```python
from build123d import *

# Parameters (mm, degrees)
SKETCH_1_R      = 2
SKETCH_1_R_2    = 5.02
SKETCH_1_R_3    = 2.05
SKETCH_1_W      = 8.2
SKETCH_1_H      = 2.2
EXTRUDE_1_DEPTH = 2
FILLET_1_R      = 1


with BuildPart() as part:
    # 草图1 → 凸台-拉伸1 (new body)
    with BuildSketch(Plane.XY):
        with BuildLine():
            Line((-38.25, 66.25), (-38.25, 62.25))
            Line((-38.25, 62.25), (-40.15, 62.25))
            Line((-40.15, 62.25), (-40.15, 59.05))
            Line((-40.15, 59.05), (-38.25, 59.05))
            Line((-38.25, 59.05), (-38.25, 55.85))
            Line((-38.25, 55.85), (-34.15, 55.85))
            Line((-34.15, 55.85), (-34.15, 59.05))
            Line((-34.15, 59.05), (-32.25, 59.05))
            Line((-32.25, 59.05), (-32.25, 62.25))
            Line((-32.25, 62.25), (-34.15, 62.25))
            Line((-34.15, 62.25), (-34.15, 66.25))
            Line((-34.15, 66.25), (-25.2, 66.25))
            Line((-25.2, 66.25), (-25.2, 70.25))
            Line((-25.2, 70.25), (-17.2, 70.25))
            Line((-17.2, 70.25), (-17.2, 66.25))
            Line((-17.2, 66.25), (-8.25, 66.25))
            Line((-8.25, 66.25), (-8.25, 62.25))
            Line((-8.25, 62.25), (-10.15, 62.25))
            Line((-10.15, 62.25), (-10.15, 59.05))
            Line((-10.15, 59.05), (-8.25, 59.05))
            Line((-8.25, 59.05), (-8.25, 55.85))
            Line((-8.25, 55.85), (-4.15, 55.85))
            Line((-4.15, 55.85), (-4.15, 59.05))
            Line((-4.15, 59.05), (-2.25, 59.05))
            Line((-2.25, 59.05), (-2.25, 62.25))
            Line((-2.25, 62.25), (-4.15, 62.25))
            Line((-4.15, 62.25), (-4.15, 66.25))
            Line((-4.15, 66.25), (4.8, 66.25))
            Line((4.8, 66.25), (4.8, 57.55))
            Line((4.8, 57.55), (53.793343317, -42.319549886))
            ThreePointArc((53.793343317, -42.319549886), (39.164608528, -74.656513398), (11.24, -52.75))
            Line((11.24, -52.75), (-94.15, 57.55))
            Line((-94.15, 57.55), (-94.15, 66.25))
            Line((-94.15, 66.25), (-85.2, 66.25))
            Line((-85.2, 66.25), (-85.2, 70.25))
            Line((-85.2, 70.25), (-77.2, 70.25))
            Line((-77.2, 70.25), (-77.2, 66.25))
            Line((-77.2, 66.25), (-68.25, 66.25))
            Line((-68.25, 66.25), (-68.25, 62.25))
            Line((-68.25, 62.25), (-70.15, 62.25))
            Line((-70.15, 62.25), (-70.15, 59.05))
            Line((-70.15, 59.05), (-68.25, 59.05))
            Line((-68.25, 59.05), (-68.25, 55.85))
            Line((-68.25, 55.85), (-64.15, 55.85))
            Line((-64.15, 55.85), (-64.15, 59.05))
            Line((-64.15, 59.05), (-62.25, 59.05))
            Line((-62.25, 59.05), (-62.25, 62.25))
            Line((-62.25, 62.25), (-64.15, 62.25))
            Line((-64.15, 62.25), (-64.15, 66.25))
            Line((-64.15, 66.25), (-55.2, 66.25))
            Line((-55.2, 66.25), (-55.2, 70.25))
            Line((-55.2, 70.25), (-47.2, 70.25))
            Line((-47.2, 70.25), (-47.2, 66.25))
            Line((-47.2, 66.25), (-38.25, 66.25))
        make_face()
        with Locations((7.098407643, -10.75)):
            Circle(SKETCH_1_R, mode=Mode.SUBTRACT)
        with Locations((33.795, -52.75)):
            Circle(SKETCH_1_R_2, mode=Mode.SUBTRACT)
        with Locations((-6.332168895, 10.336005166)):
            Circle(SKETCH_1_R_3, mode=Mode.SUBTRACT)
        with Locations((-19.762745434, 37.422010331)):
            Circle(SKETCH_1_R_3, mode=Mode.SUBTRACT)
        with Locations((-7.901592357, -10.75)):
            Rectangle(SKETCH_1_W, SKETCH_1_H, mode=Mode.SUBTRACT)
    extrude(amount=EXTRUDE_1_DEPTH)

    # 圆角1
    fillet_1_edges = [part.edges().sort_by_distance(p)[0] for p in [
        (-25.2, 70.25, 1),
        (-17.2, 70.25, 1),
        (-85.2, 70.25, 1),
        (-77.2, 70.25, 1),
        (-55.2, 70.25, 1),
        (-47.2, 70.25, 1),
    ]]
    fillet(fillet_1_edges, radius=FILLET_1_R)


solid = part.part
```
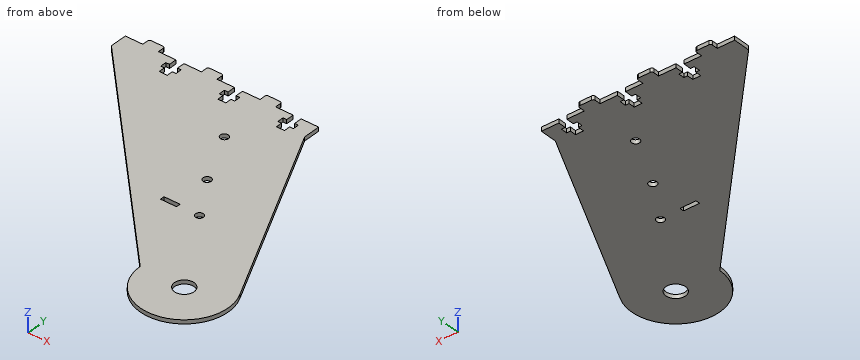
The listing builds one solid part. Answer for the finished solid, in the listing's coordinates (mm). Give positions to 0.01 mm unless a question says otherwise; leave off trailing zeros. Write each loop counter-clockwise with the first axis right and the second up, starting at its lowest first coordinate (ties: lowest second). Pieces come first, ordered by that corner, then holes. Notation, with made-up numbers: (18.25, -34) -> (43.25, -34) arc R20 cw to (43.25, -18) -> close; hole circle Ø11 at (-3, -14). An arc over 180 degrees is marked (long way). Use one line per item in the form item = value.
1) Section A-A on x = 36.5 is taken. Write down the section's boundary in (y, z).
Result:
outline = (-75.14, 0) -> (-56.98, 0) -> (-56.98, 2) -> (-75.14, 2) -> close; (-48.52, 0) -> (-7.07, 0) -> (-7.07, 2) -> (-48.52, 2) -> close
2) Section C-C on y = 25 is taken. Write down the section's boundary in (x, z).
Result:
outline = (-63.05, 0) -> (20.77, 0) -> (20.77, 2) -> (-63.05, 2) -> close
3) Straight lines are drawn through the part: probe 1 along X at (y, z) = (60.5, 1); probe 2 along Y at (x, z) = (-35.5, 0.35); probe 3 along Y at (x, z) = (31, 1.25). For each, find the intervals that lie inside material, in ascending order.
Result:
probe_1 = -94.15 to -70.15, -62.25 to -40.15, -32.25 to -10.15, -2.25 to 4.8
probe_2 = -3.83 to 55.85
probe_3 = -75.13 to -56.92, -48.58 to 4.14
4) Each of these flat-tipped pins is pushed along its axis until it touches: P1, Ø0.6, axis at y = 67.5, z = 0.5, coming from the +X side; P2, Ø1, axis at y = 60.5, z = 1, coming from the +X side; P3, Ø0.6, axis at y = 67, z = 0.5, coming from the -X side; P4, Ø8, axis at x = 33.795, y = -52.75, coming from the -Z side. Where does it stop, or does it pass through?
Result:
P1 = -17.2
P2 = 4.8
P3 = -85.2
P4 = through
5) Section D-D on x = -82 is taken. Write down the section's boundary in (y, z).
Result:
outline = (44.83, 0) -> (70.25, 0) -> (70.25, 2) -> (44.83, 2) -> close
6) Section B-B on z = 0.8 is taken. Count the separate pieces of the cut face and the enclosed holes in it, plus the area to 3 significant figures.
Result:
separate_pieces = 1
enclosed_holes = 5
area = 9,530 mm²
